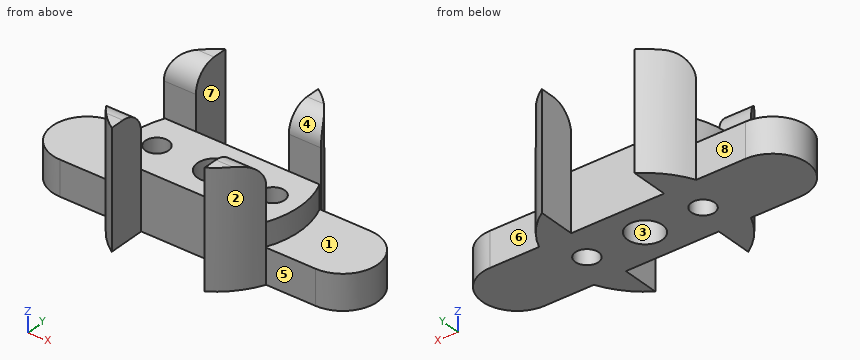
```python
from build123d import *

# Parameters (mm, degrees)
SKETCH_2_W          = 49.662427868
SKETCH_2_H          = 43.948008528
CUT_EXTRUDE_1_DEPTH = 10
SKETCH_3_R          = 1.5
SKETCH_3_R_2        = 1
CUT_EXTRUDE_2_DEPTH = 16.165750888
EXTRUDE_1_DEPTH     = 10
FILLET_1_R          = 2


with BuildPart() as part:
    # 草图1 → 旋转3 (revolve)
    with BuildSketch(Plane(origin=(0, 0, 0), x_dir=(1, 0, 0), z_dir=(0, 1, 0)), mode=Mode.PRIVATE) as revolve_3_sk:
        Polygon((0, 0), (0, 5), (20, 5), (20, 2), (7.3, 2), (7.3, 0), align=None)
    revolve(revolve_3_sk.sketch.rotate(Axis((0, 0, 0), (0, 0, 1)), 180), axis=Axis((0, 0, 0), (0, 0, 1)))

    # 草图2 → 切除-拉伸1 (cut)
    with BuildSketch(Plane.XY):
        Rectangle(SKETCH_2_W, SKETCH_2_H)
        with BuildLine():
            Line((11, -3), (-11, -3))
            ThreePointArc((-11, -3), (-14, 0), (-11, 3))
            Line((-11, 3), (11, 3))
            ThreePointArc((11, 3), (14, 0), (11, -3))
        make_face(mode=Mode.SUBTRACT)
    extrude(amount=-CUT_EXTRUDE_1_DEPTH, mode=Mode.SUBTRACT)

    # 草图3 → 切除-拉伸2 (cut, through all)
    with BuildSketch(Plane.XY):
        Circle(SKETCH_3_R)
        with Locations((5, 0)):
            Circle(SKETCH_3_R_2)
        with Locations((-5, 0)):
            Circle(SKETCH_3_R_2)
    extrude(amount=-CUT_EXTRUDE_2_DEPTH, mode=Mode.SUBTRACT)

    # 草图4 → 凸台-拉伸1 (add)
    with BuildSketch(Plane(origin=(0, 0, -5), x_dir=(-1, 0, 0), z_dir=(0, 0, -1))):
        with BuildLine():
            Line((-4, 3), (-4, 6.225752967))
            ThreePointArc((-4, 6.225752967), (-5.618771945, 4.815537543), (-6.76461381, 3))
            Line((-6.76461381, 3), (-4, 3))
        make_face()
        with BuildLine():
            ThreePointArc((6.76461381, 3), (5.618771945, 4.815537543), (4, 6.225752967))
            Line((4, 6.225752967), (4, 3))
            Line((4, 3), (6.76461381, 3))
        make_face()
        with BuildLine():
            Line((6.76461381, -3), (4, -3))
            Line((4, -3), (4, -6.225752967))
            ThreePointArc((4, -6.225752967), (5.618771945, -4.815537543), (6.76461381, -3))
        make_face()
        with BuildLine():
            Line((-4, -6.225752967), (-4, -3))
            Line((-4, -3), (-6.76461381, -3))
            ThreePointArc((-6.76461381, -3), (-5.618771945, -4.815537543), (-4, -6.225752967))
        make_face()
    extrude(amount=-EXTRUDE_1_DEPTH)

    # 圆角1
    fillet_1_edges = [part.edges().sort_by_distance(p)[0] for p in [
        (5.382306905, -3, 5),
        (5.382306905, 3, 5),
        (-5.382306905, 3, 5),
        (-5.382306905, -3, 5),
    ]]
    fillet(fillet_1_edges, radius=FILLET_1_R)


solid = part.part
```
Read the model definition and answer for the solid it produces. Units are mm, in the model's axes. Face numbers are marked on the shaded views. A direction names the side the tool comes from. Coordinates: 2 decimals unless noted, no trailing zeros. Order: outer loops, then holes, each group sorted by start corner. A loop starts at its lowest first (then second) coordinate and runs counter-clockwise, first axis right, second up. Notation, with made-up numbers: (56.25, 15) - (114.25, 15) arc R24 ccw to (114.25, 26) - close; hole circle Ø11 at (24.5, 59). An arc over 180 degrees is marked (long way). Answer as a JSON object with one key per item and string values. Group by question number.
Item 1: Section D-D (y = 4.5) is taken. Give the vertices of the cut face in (x, z), plus the area to 3 significant figures.
Item 2: Section A-A (x = -5) is taken. Give the vertices of the cut face in (y, z).
Item 3: Flat-ended cylindrical pins translate along their axes: P1, Ø3.5, axis at y = 5, z = 0.5, coming from the -X side; P2, Ø1.5, axis at x = -1.5, z = -3, coming from the +Y side; P3, Ø1.8, axis at x = -1.5, y = 1.5, coming from the +Z side; P4, Ø1.6, axis at x = -5, y = 0, coming from the +Z side. Find the tip coordinate at first contact, or state that the pin passes through.
Item 4: The mould has two halves that part along X. Classify the marked faces 1, 2 and 3: +X half, -X half, draft (parallel to the pull), parting line (faces both ways), or undercut.
Item 5: Consider probe 1 along Y at (x, z) = (0, -2.55); probe 2 along Y at (x, z) = (-5, -2.05); probe 3 along X at (y, z) = (3.25, 3). Determine where each line is inside the solid, lowest interval first. Write a range as from..to.
Item 6: Section C-C (z = -1.25) is taken. Give the vertices of the cut face in (x, y).
Item 7: A tool of negligible diameter and unlimited length cuts with its end or side. For the marked faces 4, 5, 6, 7 and 8, from which of +Z, -Z, +X, -X, +Y, -Y can it reach the whole face along a straight path? Write none if from no direction.
Item 8: Section B-B (z = 1.25) is taken. Give the vertices of the cut face in (x, y), plus the area to 3 significant figures.
Results are:
{
 "1": {"outline": "(-5.87, -5) - (-4, -5) - (-4, 4.94) - (-5.87, 4.94) - close; (4, -5) - (5.87, -5) - (5.87, 4.94) - (4, 4.94) - close", "area": "37.3 mm^2"},
 "2": {"outline": "(-5.46, -5) - (-1, -5) - (-1, 0) - (-3, 0) - (-3, 3) arc R2 ccw to (-5, 5) - (-5.46, 5) - close; (1, -5) - (5.46, -5) - (5.46, 5) - (5, 5) arc R2 ccw to (3, 3) - (3, 0) - (1, 0) - close"},
 "3": {"P1": "stops at x = -6.65", "P2": "stops at y = 3", "P3": "stops at z = 0", "P4": "passes through"},
 "4": {"face 1": "draft", "face 2": "+X half", "face 3": "undercut"},
 "5": {"probe 1": "y = -3..-1.5, 1.5..3", "probe 2": "y = -5.46..-1, 1..5.46", "probe 3": "x = -6.65..-4, 4..6.65"},
 "6": {"outline": "(-6.76, -3) arc R7.4 ccw to (-4, -6.23) - (-4, -3) - (4, -3) - (4, -6.23) arc R7.4 ccw to (6.76, -3) - (6.66, -3) arc R7.3 ccw to (6.66, 3) - (6.76, 3) arc R7.4 ccw to (4, 6.23) - (4, 3) - (-4, 3) - (-4, 6.23) arc R7.4 ccw to (-6.76, 3) - (-6.66, 3) arc R7.3 ccw to (-6.66, -3) - close; hole circle Ø2 at (-5, 0); hole circle Ø3 at (0, 0); hole circle Ø2 at (5, 0)"},
 "7": {"face 4": "+Z, +X, -X", "face 5": "+Z, -Z, +X, -Y", "face 6": "+Z, -Z, +X, +Y", "face 7": "+Z, -Z, +Y", "face 8": "+Z, -Z, -X, +Y"},
 "8": {"outline": "(-6.76, -3) arc R7.4 ccw to (-4, -6.23) - (-4, -3) - close; (-6.76, 3) - (-4, 3) - (-4, 6.23) arc R7.4 ccw to start; (4, -6.23) arc R7.4 ccw to (6.76, -3) - (4, -3) - close; (4, 3) - (6.76, 3) arc R7.4 ccw to (4, 6.23) - close", "area": "21.4 mm^2"}
}
